Autodesk Inventor part; units mm, degrees
ref_plane "YZ Plane" through (0, 0, 0) normal (1, 0, 0) x (0, 1, 0)
ref_plane "XZ Plane" through (0, 0, 0) normal (0, 1, 0) x (-1, 0, 0)
ref_plane "XY Plane" through (0, 0, 0) normal (0, 0, 1) x (1, 0, 0)
sketch "Sketch1" plane through (0, 0, 0) normal (0, 0, 1) x (1, 0, 0)
  line L0 (-23.2495, 10.1907) -> (98.6705, 10.1907)
  line L1 (98.6705, 10.1907) -> (98.6705, -66.0093)
  line L2 (98.6705, -66.0093) -> (-23.2495, -66.0093)
  line L3 (-23.2495, -66.0093) -> (-23.2495, 10.1907)
  point P0 (0, 0)
  dimension "d0" = 121.92
  dimension "d1" = 76.2
extrude "Extrusion1" add sketch "Sketch1" along normal blind 1.5875
sketch "Sketch2" plane through (0, 0, 1.5875) normal (0, 0, 1) x (1, 0, 0)
  circle A0 centre (-13.3114, -27.9093) radius 2
  circle A1 centre (3.1346, -27.9093) radius 2
  circle A2 centre (19.5806, -27.9093) radius 2
  circle A3 centre (36.0266, -27.9093) radius 2
  circle A4 centre (68.9186, -27.9093) radius 2
  circle A5 centre (85.3646, -27.9093) radius 2
  line L0 (98.6705, -66.0093) -> (98.6705, 10.1907)
  line L1 (68.9186, -27.9093) -> (51.2881, -27.9093) construction
  circle A6 centre (52.4726, -27.9093) radius 2
  point P0 (0, 0)
  dimension "d4" = 4
  dimension "d5" = 4
  dimension "d6" = 4
  dimension "d7" = 4
  dimension "d9" = 4
  dimension "d10" = 4
  dimension "d11" = 12.446
  dimension "d12" = 12.446
  dimension "d13" = 12.446
  dimension "d18" = 4
  dimension "d20" = 12.446
  dimension "d21" = 12.446
  dimension "d22" = 12.446
extrude "Extrusion2" cut sketch "Sketch2" against normal blind 1.5875
properties part number "topgearbase"
Check sheet for the modelled part. Datum: model origin and axes. Units: mm. Coordinates: 2 decimals unless noted, no trailing zeros.
Item 1: Scan lines: probe 1 along Y at (x, z) = (-13.5, 0.15); probe 2 along Y at (x, z) = (35, 0.75). Record each from-to range of solid material in increasing order.
Numbers:
probe 1: y = -66.01 to -29.9, -25.92 to 10.19
probe 2: y = -66.01 to -29.63, -26.19 to 10.19
Item 2: Depth check by flat-ended pin: pin 1 Ø6.5 at (x, y) = (85.36, -27.91) entering from +Z. Enter the tip coordinate at first touch or a pass-through.
Numbers:
pin 1: stops at z = 1.59
Item 3: Mould release check, pull along X, two halves, no side actions. Record for faces 1 (the face through (2.874, -25.926, 0.805)), 2 (the face through (37, -19, 0)): released by +X, released by -X, zero draft, split by the parting line, or undercut.
Numbers:
face 1: undercut
face 2: zero draft
